For this review, take the finished solid that the model builds, in its own axes (mm). A direction names the side the tool comes from. Give positions to 0.01 mm unless a question says otherwise; leave off trailing zeros. Write each loop counter-clockwise with the first axis right and the second up, starting at its lowest first coordinate (ties: lowest second). Pieces come first, ordered by that corner, then holes.
Q1. We need section C-C (x = 13). Write out the cut boundary in (y, z).
Q2. Machinability: for faces 1 (the cylindrical face through (-6.876, 27.227, -8.967)), 2 (the cylindrical face through (-5.3, 48.52, 13.61)), 3 (the flat face through (2.5, 25, -7)), which of the approach directions +Z, -Z, +X, -X, +Y, -Y give a long, thin tool a straight path to every point of the face, cutting with its end or side? Answer none if there is none.
Q3. For line 1 (X direction, y = 18, z = 0); line 2 (Y direction, x = -10.5, z = 9.5); line 3 (Z direction, x = 4, y = 35), list the stretches that pass through material, from the lowest coordinate up.
Q4. We need section D-D (x = -5.5). Write out the cut boundary in (y, z).
Q5. Insertion check: P1, Ø4, axis at x = 0.5, y = 20.5, coming from the +Z side; P2, Ø5, axis at x = 8, y = 37.5, coming from the -Z side; P3, Ø1.5, axis at x = -6.5, y = 43.5, coming from the -Z side; P4, Ø6, axis at x = 1.5, z = 6, coming from the -Y side. Each pin has a flat end and moves straight along its axis. Give the tip position at first contact, or say it passes through.
Q6. We need section A-A (y = 5). Write out the cut boundary in (x, z).
Q7. We need section B-B (z = -1). Write out the cut boundary in (x, y), then the cut area to 3 significant figures.
Q8. Mouldability with a two-part tool opening along Y and no side actions: class faces 4 (the flat face through (-3, 50.089, 6)), 5 (the flat face through (-10, 8, -6)), 6 (the flat face through (-2.5, 25, -7)), 7 (the flat face through (5, 47, -11)) as released by +Y, released by -Y, zero draft, split by the parting line, or undercut.
```python
from build123d import *

# Parameters (mm, degrees)
SKETCH1_R           = 15.3
BOSS_EXTRUDE1_DEPTH = 8
SKETCH2_R           = 11.3
BOSS_EXTRUDE2_DEPTH = 39
SKETCH3_R           = 15.3
BOSS_EXTRUDE3_DEPTH = 3.088651712
CUT_EXTRUDE4_DEPTH  = 51


with BuildPart() as part:
    # Sketch1 → Boss-Extrude1 (new body)
    with BuildSketch(Plane(origin=(0, 0, 0), x_dir=(1, 0, 0), z_dir=(0, 1, 0))):
        with Locations(Location((0, 0, 0), (0, 0, 270))):
            Circle(SKETCH1_R)
    extrude(amount=BOSS_EXTRUDE1_DEPTH)

    # Sketch2 → Boss-Extrude2 (add)
    with BuildSketch(Plane(origin=(0, 8, 0), x_dir=(1, 0, 0), z_dir=(0, 1, 0))):
        with Locations(Location((0, 0, 0), (0, 0, 270))):
            Circle(SKETCH2_R)
    extrude(amount=BOSS_EXTRUDE2_DEPTH)

    # Sketch3 → Boss-Extrude3 (add)
    with BuildSketch(Plane(origin=(0, 47, 0), x_dir=(1, 0, 0), z_dir=(0, 1, 0))):
        with Locations(Location((0.559173948, 0.524225576, 0), (0, 0, 270))):
            Circle(SKETCH3_R)
    extrude(amount=BOSS_EXTRUDE3_DEPTH)

    # Sketch6 → Cut-Extrude4 (cut)
    with BuildSketch(Plane(origin=(0, 50.088651712, 0), x_dir=(1, 0, 0), z_dir=(0, 1, 0))):
        with BuildLine():
            Line((-2.5, 8.9), (2.5, 8.9))
            Line((2.5, 8.9), (2.5, 6))
            ThreePointArc((2.5, 6), (0, -6.5), (-2.5, 6))
            Line((-2.5, 6), (-2.5, 8.9))
        make_face()
    extrude(amount=-CUT_EXTRUDE4_DEPTH, mode=Mode.SUBTRACT)


solid = part.part
```
Computed:
1. outline: (0, -8.07) - (8, -8.07) - (8, 8.07) - (0, 8.07) - close; (47, -9.43) - (50.09, -9.43) - (50.09, 8.38) - (47, 8.38) - close
2. face 1: none
2. face 2: +Y
2. face 3: +Y, -Y
3. line 1: x = -11.3 to -6.5, 6.5 to 11.3
3. line 2: y = 0 to 8, 47 to 50.09
3. line 3: z = -10.57 to -5.12, 5.12 to 10.57
4. outline: (0, -14.28) - (8, -14.28) - (8, -9.87) - (47, -9.87) - (47, -14.57) - (50.09, -14.57) - (50.09, -3.46) - (0, -3.46) - close; (0, 3.46) - (50.09, 3.46) - (50.09, 13.52) - (47, 13.52) - (47, 9.87) - (8, 9.87) - (8, 14.28) - (0, 14.28) - close
5. P1: stops at z = 11.3
5. P2: stops at z = -9.87
5. P3: stops at z = -9.73
5. P4: stops at y = 0
6. outline: circle Ø30.6 at (0, 0); hole (-2.5, -8.9) - (2.5, -8.9) - (2.5, -6) arc R6.5 ccw (long way) to (-2.5, -6) - close
7. outline: (-15.27, 0) - (-6.42, 0) - (-6.42, 50.09) - (-14.73, 50.09) - (-14.73, 47) - (-11.26, 47) - (-11.26, 8) - (-15.27, 8) - close; (6.42, 0) - (15.27, 0) - (15.27, 8) - (11.26, 8) - (11.26, 47) - (15.85, 47) - (15.85, 50.09) - (6.42, 50.09) - close
7. area: 573 mm2
8. face 4: released by +Y
8. face 5: undercut
8. face 6: zero draft
8. face 7: undercut
